Input: part model. Units: mm. Frame: model coordinates. Coordinates: 2 decimals unless noted, no trailing zeros. Order: outer loops, then holes, each group sorted by start corner. A loop starts at its lowest first (then second) coordinate and runs counter-clockwise, first axis right, second up. Notation, with made-up numbers: (15.25, -0.5) -> (61.25, -0.5) arc R19 ccw to (61.25, 10.5) -> close; hole circle Ø8 at (73.5, 81). An arc over 180 degrees is marked (long way). Use CSV: the item, a comma, the result in double quotes. Start each with the question number.
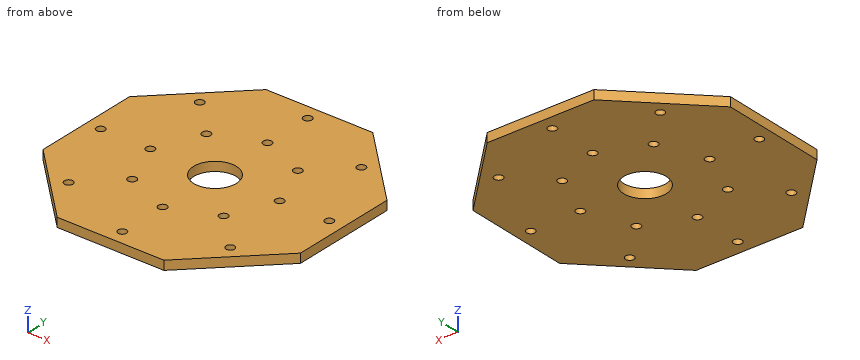
```python
from build123d import *

# Parameters (mm, degrees)
F0_R     = 1.4
F0_R_2   = 7
F1_DEPTH = 3


with BuildPart() as f1:
    # F0 (on Top) → F1 (new body)
    with BuildSketch(Plane.XY):
        Polygon((17.5, 42.248737), (-17.5, 42.248737), (-42.248737, 17.5), (-42.248737, -17.5), (-17.5, -42.248737), (17.5, -42.248737), (42.248737, -17.5), (42.248737, 17.5), align=None)
        with Locations((-26.516504, -26.516504)):
            Circle(F0_R, mode=Mode.SUBTRACT)
        with Locations((-37.5, 0)):
            Circle(F0_R, mode=Mode.SUBTRACT)
        with Locations((-21.213203, 0)):
            Circle(F0_R, mode=Mode.SUBTRACT)
        with Locations((-15, -15)):
            Circle(F0_R, mode=Mode.SUBTRACT)
        with Locations((0, -37.5)):
            Circle(F0_R, mode=Mode.SUBTRACT)
        with Locations((0, -21.213203)):
            Circle(F0_R, mode=Mode.SUBTRACT)
        with Locations((26.516504, -26.516504)):
            Circle(F0_R, mode=Mode.SUBTRACT)
        with Locations((15, -15)):
            Circle(F0_R, mode=Mode.SUBTRACT)
        Circle(F0_R_2, mode=Mode.SUBTRACT)
        with Locations((21.213203, 0)):
            Circle(F0_R, mode=Mode.SUBTRACT)
        with Locations((37.5, 0)):
            Circle(F0_R, mode=Mode.SUBTRACT)
        with Locations((-15, 15)):
            Circle(F0_R, mode=Mode.SUBTRACT)
        with Locations((-26.516504, 26.516504)):
            Circle(F0_R, mode=Mode.SUBTRACT)
        with Locations((15, 15)):
            Circle(F0_R, mode=Mode.SUBTRACT)
        with Locations((0, 21.213203)):
            Circle(F0_R, mode=Mode.SUBTRACT)
        with Locations((0, 37.5)):
            Circle(F0_R, mode=Mode.SUBTRACT)
        with Locations((26.516504, 26.516504)):
            Circle(F0_R, mode=Mode.SUBTRACT)
    extrude(amount=F1_DEPTH)


solid = f1.part
```
1. Section D-D on y = -37.5. Return loops of the section in (x, z).
2. Section A-A on x = 0. Return loops of the section in (y, z).
3. Contact query for flat-ended pins moving along their axis: P1, Ø2, axis at x = 26.52, y = 26.52, coming from the +Z side; P2, Ø1, axis at x = 28, z = 1.5, coming from the +Y side. Output: stop coordinate, or through.
4. Material intervals for line 1 along Y through (x, z) = (0, 1.3); line 2 along Y through (x, z) = (-15, 1.4); line 3 along Y through (x, z) = (-14.5, 2.55), sorted ascending.
5. Section B-B on x = 15. Return loops of the section in (y, z), then the cut area to 3 significant figures.
Values follow:
1,outline,"(-22.25, 0) -> (-1.4, 0) -> (-1.4, 3) -> (-22.25, 3) -> close; (1.4, 0) -> (22.25, 0) -> (22.25, 3) -> (1.4, 3) -> close"
2,outline,"(-42.25, 0) -> (-38.9, 0) -> (-38.9, 3) -> (-42.25, 3) -> close; (-36.1, 0) -> (-22.61, 0) -> (-22.61, 3) -> (-36.1, 3) -> close; (-19.81, 0) -> (-7, 0) -> (-7, 3) -> (-19.81, 3) -> close; (7, 0) -> (19.81, 0) -> (19.81, 3) -> (7, 3) -> close; (22.61, 0) -> (36.1, 0) -> (36.1, 3) -> (22.61, 3) -> close; (38.9, 0) -> (42.25, 0) -> (42.25, 3) -> (38.9, 3) -> close"
3,P1,"passes through"
3,P2,"stops at y = 32.25"
4,line 1,"y = -42.25 to -38.9, -36.1 to -22.61, -19.81 to -7, 7 to 19.81, 22.61 to 36.1, 38.9 to 42.25"
4,line 2,"y = -42.25 to -16.4, -13.6 to 13.6, 16.4 to 42.25"
4,line 3,"y = -42.25 to -16.31, -13.69 to 13.69, 16.31 to 42.25"
5,outline,"(-42.25, 0) -> (-16.4, 0) -> (-16.4, 3) -> (-42.25, 3) -> close; (-13.6, 0) -> (13.6, 0) -> (13.6, 3) -> (-13.6, 3) -> close; (16.4, 0) -> (42.25, 0) -> (42.25, 3) -> (16.4, 3) -> close"
5,area,"237 mm2"
